Geometry check sheet. Reference: the model listing, model coordinates, mm. Give positions to 0.01 mm unless a question says otherwise; leave off trailing zeros. Loops run counter-clockwise (first coordinate to the right, second up) from the corner with the lowest first, then second, coordinate; pieces in that order, holes last. Notation, with made-up numbers: (45, -37) -> (70, -37) arc R18 ccw to (70, -13) -> close; hole circle Ø1 at (-1, 46.5). An arc over 180 degrees is marked (long way). Write item = value, one per line. Start each with the question number.
```python
from build123d import *

# Parameters (mm, degrees)
SKETCH1_R                   = 25.4
BOSS_EXTRUDE1_DEPTH         = 12.7
FILLET1_R                   = 2.54
FILLET2_R                   = 2.54
F_1_4_0_25_DIAMETER_HOLE1_D = 6.35


with BuildPart() as part:
    # Sketch1 → Boss-Extrude1 (new body)
    with BuildSketch(Plane.XY):
        with Locations((-30.291010944, 15.918155424)):
            Circle(SKETCH1_R)
    extrude(amount=BOSS_EXTRUDE1_DEPTH)

    # Fillet1
    fillet1_edges = [part.edges().sort_by_distance(p)[0] for p in [
        (-55.691010944, 15.918155424, 12.7),
    ]]
    fillet(fillet1_edges, radius=FILLET1_R)

    # Fillet2
    fillet2_edges = [part.edges().sort_by_distance(p)[0] for p in [
        (-55.691010944, 15.918155424, 0),
    ]]
    fillet(fillet2_edges, radius=FILLET2_R)

    # 1/4 (0.25) Diameter Hole1 (through all)
    with Locations(Plane(origin=(0, 0, 0), x_dir=(-1, 0, 0), z_dir=(0, 0, -1))):
        with Locations((28.50138728, 13.874510617)):
            Hole(F_1_4_0_25_DIAMETER_HOLE1_D / 2)


solid = part.part
```
1) Draft check along X on faces 1 (the cylindrical face through (-6.064, 23.548, 6.297)), 2 (the cylindrical face through (-31.02, 11.94, 6.44)), 3 (the flat face through (-31, 11, 12.7)). Enter one of: released by +X, released by -X, zero draft, split by the parting line, or undercut.
2) Depth check by flat-ended pin: pin 1 Ø5 at (x, z) = (-11.5, 7.5) entering from +Y; pin 2 Ø6 at (x, z) = (-45, 7) entering from +Y; pin 3 Ø4 at (y, z) = (27.5, 6.5) entering from -X. Enter the tip coordinate at first touch or a pass-through.
3) Section check A-A (z = 3.25). Enter the section's corners in (x, y) (3 decimals), plus the area to 3 significant figures.
4) Thickness scan on line 1 (Y direction, x = -27.5, z = 2.25); line 2 (Y direction, x = -28.5, z = 10.5); line 3 (X direction, y = 13, z = 2.5). Record the ranges inside material, lowest first.
5) Section check B-B (z = 11.25). Enter the section's corners in (x, y) (3 decimals), plus the area to 3 significant figures.
Check result:
q1.face_1 = split by the parting line
q1.face_2 = undercut
q1.face_3 = zero draft
q2.pin_1 = 35.41
q2.pin_2 = 38.46
q2.pin_3 = -53.81
q3.outline = circle Ø50.8 at (-30.291, 15.918); hole circle Ø6.35 at (-28.501, 13.875)
q3.area = 2,000 mm2
q4.line_1 = -9.31 to 10.86, 16.89 to 41.15
q4.line_2 = -9.4 to 10.7, 17.05 to 41.23
q4.line_3 = -55.52 to -31.55, -25.45 to -5.06
q5.outline = circle Ø50.308 at (-30.291, 15.918); hole circle Ø6.35 at (-28.501, 13.875)
q5.area = 1,960 mm2
